```python
from build123d import *

# Parameters (mm, degrees)
SKETCH1_R           = 20
BOSS_EXTRUDE3_DEPTH = 10


with BuildPart() as part:
    # Sketch1 → Boss-Extrude3 (new body)
    with BuildSketch(Plane(origin=(0, 0, 0), x_dir=(1, 0, 0), z_dir=(0, 1, 0))):
        with BuildLine():
            Line((-80, 50), (80, 50))
            ThreePointArc((80, 50), (94.142135624, 44.142135624), (100, 30))
            Line((100, 30), (100, -50))
            Line((100, -50), (-100, -50))
            Line((-100, -50), (-100, 30))
            ThreePointArc((-100, 30), (-94.142135624, 44.142135624), (-80, 50))
        make_face()
        with Locations(Location((0, 26.715686275, 0), (0, 0, 270))):
            Circle(SKETCH1_R, mode=Mode.SUBTRACT)
        with Locations(Location((73.039215686, 0, 0), (0, 0, 270))):
            Circle(SKETCH1_R, mode=Mode.SUBTRACT)
        with Locations(Location((-67.156862745, 0, 0), (0, 0, 270))):
            Circle(SKETCH1_R, mode=Mode.SUBTRACT)
    extrude(amount=BOSS_EXTRUDE3_DEPTH)


solid = part.part
```
Verification items for the finished model (mm, model axes). Give positions to 0.01 mm unless a question says otherwise; leave off trailing zeros. Order: outer loops, then holes, each group sorted by start corner. A loop starts at its lowest first (then second) coordinate and runs counter-clockwise, first axis right, second up. Notation, with made-up numbers: M 17.25,24 L 21.25,24 A19 cw 21.25,29 Z; hole C 32,54.25 d1. An arc over 180 degrees is marked long. Answer in a Markdown table with one row per item. Add a question column.
Item 1: Section check D-D, the plane y = 1.75. Enter the section's corners in (x, z).
Item 2: Mould release check, pull along X, two halves, no side actions. Record for faces 1 (the cylindrical face through (92.87, 4.93, -2.6)), 2 (the cylindrical face through (93.986, 4.93, -44.297)), 3 (the flat face through (-1, 5, -50)): released by +X, released by -X, zero draft, split by the parting line, or undercut.
Item 3: Section check C-C, the plane z = -23. Enter the section's corners in (x, y).
Item 4: Section check B-B, the plane x = 0. Enter the section's corners in (y, z).
Item 5: Section check A-A, the plane z = 0. Enter the section's corners in (x, y), and give its area (3 significant figures).
Item 6: Scan lines: probe 1 along X at (y, z) = (5.75, -12); probe 2 along X at (y, z) = (2.25, -27); probe 3 along Z at (x, y) = (-49, 6.75). Record each from-to range of solid material in increasing order. Write a range as from..to.
Filled sheet:
| question | item | result |
|---|---|---|
| 1 | outline | M -100,-30 A20 ccw -80,-50 L 80,-50 A20 ccw 100,-30 L 100,50 L -100,50 Z; hole C -67.16,0 d40; hole C 0,-26.72 d40; hole C 73.04,0 d40 |
| 2 | face 1 | undercut |
| 2 | face 2 | released by +X |
| 2 | face 3 | zero draft |
| 3 | outline | M -100,0 L -19.65,0 L -19.65,10 L -100,10 Z; M 19.65,0 L 100,0 L 100,10 L 19.65,10 Z |
| 4 | outline | M 0,-50 L 10,-50 L 10,-46.72 L 0,-46.72 Z; M 0,-6.72 L 10,-6.72 L 10,50 L 0,50 Z |
| 5 | outline | M -100,0 L -87.16,0 L -87.16,10 L -100,10 Z; M -47.16,0 L 53.04,0 L 53.04,10 L -47.16,10 Z; M 93.04,0 L 100,0 L 100,10 L 93.04,10 Z |
| 5 | area | 1,200 mm^2 |
| 6 | probe 1 | x = -100..-83.16, -51.16..-13.54, 13.54..57.04, 89.04..100 |
| 6 | probe 2 | x = -100..-20, 20..100 |
| 6 | probe 3 | z = -50..-8.39, 8.39..50 |
